Could you check a few things on this model? Use its own coordinates, in mm. Face numbers are marked on the shaded views. Give positions to 0.01 mm unless a question says otherwise; leave off trailing zeros. Loops run counter-clockwise (first coordinate to the right, second up) from the corner with the lowest first, then second, coordinate; pieces in that order, holes last. Notation, with made-up numbers: (65.25, 35.5) - (119.25, 35.5) arc R30 ccw to (119.25, 68.5) - close; hole circle Ø7 at (35.5, 32). An arc over 180 degrees is marked (long way). Write each question's results on one line, items separated by ' | '. Start each with the question number.
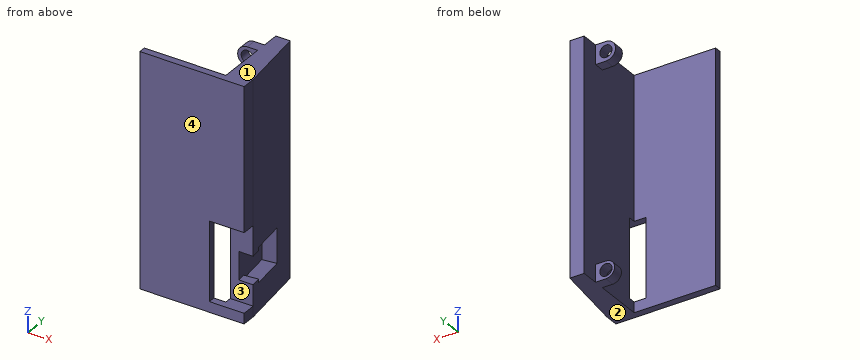
```python
from build123d import *

# Parameters (mm, degrees)
EXTRUDE_1_DEPTH     = 3
EXTRUDE_2_DEPTH     = 66.63
CUT_EXTRUDE_1_DEPTH = 69.53372087
SKETCH_4_W          = 8
SKETCH_4_H          = 3
CUT_EXTRUDE_2_DEPTH = 10
SKETCH_5_W          = 6.574056315
SKETCH_5_H          = 41
SKETCH_5_H_2        = 3
EXTRUDE_3_DEPTH     = 2
SKETCH_6_W          = 20
SKETCH_6_H          = 22.63
SKETCH_6_W_2        = 30
SKETCH_6_H_2        = 41
SKETCH_6_H_3        = 3
EXTRUDE_4_DEPTH     = 2


with BuildPart() as part:
    # 草图1 → 凸台-拉伸1 (new body)
    with BuildSketch(Plane(origin=(0, 0, 0), x_dir=(1, 0, 0), z_dir=(0, 1, 0))):
        with BuildLine():
            ThreePointArc((2.75, -61.38), (1.944543648, -59.435456352), (0, -58.63))
            Line((0, -58.63), (0, -59.63))
            ThreePointArc((0, -59.63), (1.237436867, -60.142563133), (1.75, -61.38))
            ThreePointArc((1.75, -61.38), (1.237436867, -62.617436867), (0, -63.13))
            Line((0, -63.13), (0, -64.13))
            ThreePointArc((0, -64.13), (1.944543648, -63.324543648), (2.75, -61.38))
        make_face()
        with BuildLine():
            Line((0, -59.63), (0, -58.63))
            ThreePointArc((0, -58.63), (-2.75, -61.38), (0, -64.13))
            Line((0, -64.13), (0, -63.13))
            ThreePointArc((0, -63.13), (-1.75, -61.38), (0, -59.63))
        make_face()
        with BuildLine():
            Line((5, -58.63), (0, -58.63))
            ThreePointArc((0, -58.63), (1.944543648, -59.435456352), (2.75, -61.38))
            ThreePointArc((2.75, -61.38), (1.944543648, -63.324543648), (0, -64.13))
            Line((0, -64.13), (5, -64.13))
            Line((5, -64.13), (5, -58.63))
        make_face()
        Polygon((5, -2.5), (5, -58.63), (5, -64.13), (8, -64.13), (8, 2.5), (5, 2.5), align=None)
        with BuildLine():
            ThreePointArc((0, 2.5), (-2.5, 0), (0, -2.5))
            Line((0, -2.5), (0, -1.75))
            ThreePointArc((0, -1.75), (-1.75, 0), (0, 1.75))
            Line((0, 1.75), (0, 2.5))
        make_face()
        with BuildLine():
            Line((0, -1.75), (0, -2.5))
            ThreePointArc((0, -2.5), (1.767766953, -1.767766953), (2.5, 0))
            ThreePointArc((2.5, 0), (1.767766953, 1.767766953), (0, 2.5))
            Line((0, 2.5), (0, 1.75))
            ThreePointArc((0, 1.75), (1.237436867, 1.237436867), (1.75, 0))
            ThreePointArc((1.75, 0), (1.237436867, -1.237436867), (0, -1.75))
        make_face()
        with BuildLine():
            Line((0, -2.5), (5, -2.5))
            Line((5, -2.5), (5, 2.5))
            Line((5, 2.5), (0, 2.5))
            ThreePointArc((0, 2.5), (1.767766953, 1.767766953), (2.5, 0))
            ThreePointArc((2.5, 0), (1.767766953, -1.767766953), (0, -2.5))
        make_face()
    extrude(amount=EXTRUDE_1_DEPTH)

    # 草图2 → 凸台-拉伸2 (add, through all)
    with BuildSketch(Plane.XY.offset(64.13)):
        Polygon((3, 3), (8, 3), (7.118365096, 8), (3, 8), align=None)
        Polygon((3, -12), (3, 3), (8, 3), (10.644904711, -12), align=None)
    extrude(amount=-EXTRUDE_2_DEPTH)

    # 草图3 → 切除-拉伸1 (cut, through all)
    with BuildSketch(Plane.XY.offset(64.13)):
        Polygon((10.468020954, -13.888439464), (9.574056315, -12), (7.118365096, 8), (7.997986879, 8.163017845), (13.179200704, -12.892022974), align=None)
    extrude(amount=-CUT_EXTRUDE_1_DEPTH, mode=Mode.SUBTRACT)

    # 草图4 → 切除-拉伸2 (cut)
    with BuildSketch(Plane(origin=(3.923131172, 0.481699938, 0), x_dir=(0, 0, -1), z_dir=(0.9925461516413224, 0.12186934340514417, 0))):
        Polygon((-5.5, -10.077337776), (-5.5, -0.077337776), (-15.5, -0.077337776), (-15.5, -10.077337776), (-14.5, -10.077337776), (-14.5, -7.077337776), (-6.5, -7.077337776), (-6.5, -10.077337776), align=None)
        with Locations((-10.5, -8.577337776)):
            Rectangle(SKETCH_4_W, SKETCH_4_H)
        with Locations((-10.5, -11.577337776)):
            Rectangle(SKETCH_4_W, SKETCH_4_H)
    extrude(amount=CUT_EXTRUDE_2_DEPTH, mode=Mode.SUBTRACT)

    # 草图5 → 凸台-拉伸3 (add)
    with BuildSketch(Plane(origin=(0, -12, 0), x_dir=(-1, 0, 0), z_dir=(0, -1, 0))):
        with Locations((-6.287028157, -43.63)):
            Rectangle(SKETCH_5_W, SKETCH_5_H)
        with Locations((-6.287028157, 1)):
            Rectangle(SKETCH_5_W, SKETCH_5_H_2)
    extrude(amount=EXTRUDE_3_DEPTH)

    # 草图6 → 凸台-拉伸4 (add)
    with BuildSketch(Plane(origin=(0, -14, 0), x_dir=(-1, 0, 0), z_dir=(0, -1, 0))):
        with Locations((10.425943685, -11.815)):
            Rectangle(SKETCH_6_W, SKETCH_6_H)
        with Locations((5.425943685, -43.63)):
            Rectangle(SKETCH_6_W_2, SKETCH_6_H_2)
        with Locations((5.425943685, 1)):
            Rectangle(SKETCH_6_W_2, SKETCH_6_H_3)
    extrude(amount=EXTRUDE_4_DEPTH)


solid = part.part
```
Q1. I want a section at C-C, the plane y = -7. List the corners of the cut face in (x, z) for me.
Q2. I'm going to push flat-ended pins straight in: pin 1 Ø12 at (x, z) = (-10, 49) entering from +Y; pin 2 Ø2 at (x, z) = (5.5, 9.5) entering from -Y; pin 3 Ø6 at (x, z) = (0.5, 62.5) entering from +Y; pin 4 Ø3 at (x, y) = (-8, -11.5) entering from +Z. Where does each tip first touch, or does it pass through?
Q3. If we mould it in two halves opening along Z, with no side actions, what happens to the marked faces 1, 2, 3 and 4? For each: +Z half, -Z half, draft (parallel to the pull), parting line (faces both ways), or undercut.
Q4. I need wall thicknesses on L1, parallel to Y at x = -15.5, z = 43; L2, parallel to X at y = 1, z = 30.5; L3, parallel to Z at x = 8.25, y = -13. Which ranges of each line are inside material? Lowest first, please. Write a range as from..to.
Q5. I want a section at A-A, the plane z = 39. List the corners of the cut face in (x, y) for me, then the cut area to 3 significant figures.
Q6. I want a section at D-D, the plane y = 5. List the corners of the cut face in (x, z) for me.
Q7. I want a section at B-B, the plane x = -16. List the corners of the cut face in (y, z) for me.
Conclusion:
1) outline: (3, -2.5) - (8.96, -2.5) - (8.96, 5.5) - (4.84, 5.5) - (4.84, 15.5) - (8.96, 15.5) - (8.96, 64.13) - (3, 64.13) - close
2) pin 1: y = -14 | pin 2: y = -12 | pin 3: y = 8 | pin 4: through
3) face 1: +Z half | face 2: -Z half | face 3: undercut | face 4: draft
4) L1: -16..-14 | L2: 3..7.98 | L3: -2.5..0.5, 23.13..64.13
5) outline: (-20.43, -16) - (9.57, -16) - (9.57, -12) - (7.12, 8) - (3, 8) - (3, -14) - (-20.43, -14) - close | area: 180 mm^2
6) outline: (3, -2.5) - (7.49, -2.5) - (7.49, 64.13) - (3, 64.13) - close
7) outline: (-16, -2.5) - (-14, -2.5) - (-14, 64.13) - (-16, 64.13) - close
